Print and shaded views of the part. All mm, measured from the part's lowest x, y and z. Give positions to 0.01 mm unless a question says otherwise; leave off trailing zeros. Order: outer loops, then holes, each group sorted by start corner. A loop starts at its lowest first (then second) coordinate and runs counter-clockwise, first axis right, second up. Notation, with made-up numbers: (-17.75, 60.5) -> (-11.75, 60.5) arc R31 ccw to (-11.75, 92.5) -> close; hole circle Ø11 at (52, -20.75). An arc over 180 degrees is marked (long way). One line per question, with ' | ' between items. Start each with the question number.
(1) Pin check, flat tips, straight feed: pin 1 Ø3 at (x, z) = (14.5, 25.5) entering from -Y; pin 2 Ø1.2 at (y, z) = (1.5, 38) entering from -X. Stop position of each tip, or through.
(2) Cut at C-C (x = 4.5). Give the cut face in (y, z).
(3) Drill centre lines: L1, parallel to Z at x = 4.5, y = 2.65; L2, parallel to X at y = 1.3, z = 11; L3, parallel to X at y = 0.4, z = 4. Where is each one in solid material? Low to high. Write a range as from..to.
(4) Cut at A-A (z = 5). Give the cut face in (x, y), then the cut area to 3 significant figures.
(5) Cut at D-D (z = 26). Give the cut face in (x, y).
(6) Cut at B-B (y = 2.6). Give the cut face in (x, z), then the cut area to 3 significant figures.
(7) Pull direction Z, two halves, no side cores. Call the marked faces 1, 2 and 3: +Z half, -Z half, draft (parallel to the pull), parting line (faces both ways), or undercut.
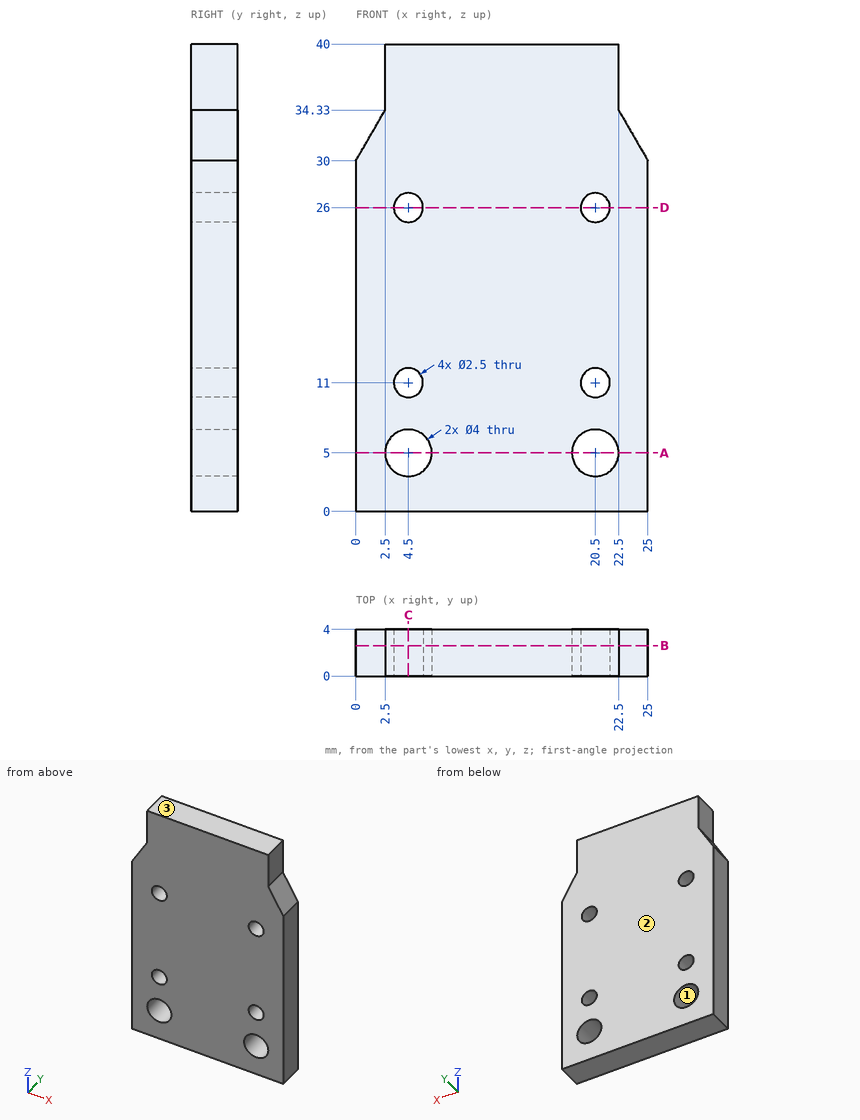
Result set:
1) pin 1: stops at y = 0 | pin 2: stops at x = 2.5
2) outline: (0, 0) -> (4, 0) -> (4, 3) -> (0, 3) -> close; (0, 7) -> (4, 7) -> (4, 9.75) -> (0, 9.75) -> close; (0, 12.25) -> (4, 12.25) -> (4, 24.75) -> (0, 24.75) -> close; (0, 27.25) -> (4, 27.25) -> (4, 40) -> (0, 40) -> close
3) L1: z = 0..3, 7..9.75, 12.25..24.75, 27.25..40 | L2: x = 0..3.25, 5.75..19.25, 21.75..25 | L3: x = 0..2.77, 6.23..18.77, 22.23..25
4) outline: (0, 0) -> (2.5, 0) -> (2.5, 4) -> (0, 4) -> close; (6.5, 0) -> (18.5, 0) -> (18.5, 4) -> (6.5, 4) -> close; (22.5, 0) -> (25, 0) -> (25, 4) -> (22.5, 4) -> close | area: 68.0 mm2
5) outline: (0, 0) -> (3.25, 0) -> (3.25, 4) -> (0, 4) -> close; (5.75, 0) -> (19.25, 0) -> (19.25, 4) -> (5.75, 4) -> close; (21.75, 0) -> (25, 0) -> (25, 4) -> (21.75, 4) -> close
6) outline: (0, 0) -> (25, 0) -> (25, 30) -> (22.5, 34.33) -> (22.5, 40) -> (2.5, 40) -> (2.5, 34.33) -> (0, 30) -> close; hole circle Ø4 at (4.5, 5); hole circle Ø2.5 at (4.5, 11); hole circle Ø2.5 at (4.5, 26); hole circle Ø4 at (20.5, 5); hole circle Ø2.5 at (20.5, 11); hole circle Ø2.5 at (20.5, 26) | area: 916 mm2
7) face 1: undercut | face 2: draft | face 3: +Z half
